Could you check a few things on this model? Use its own coordinates, in mm. Face numbers are marked on the shaded views. A direction names the side the tool comes from. Give positions to 0.01 mm unless a question says otherwise; leave off trailing zeros. Write each loop counter-clockwise with the first axis right and the second up, starting at its lowest first coordinate (ties: lowest second). Pieces come first, ordered by that corner, then holes. Notation, with made-up numbers: M -23.75,39.25 L 28.25,39.25 A9 ccw 28.25,47.25 Z; hole C 69.5,-6 d1. An arc over 180 degrees is marked long. Use one line per item in the form item = value.
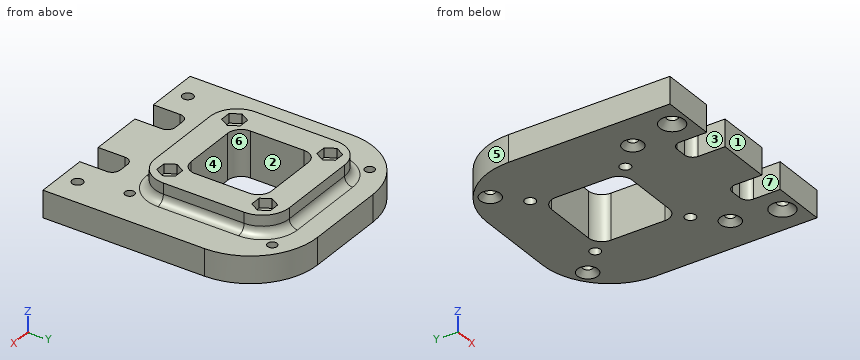
Autodesk Inventor part; units mm, degrees
ref_plane "YZ Plane" through (0, 0, 0) normal (1, 0, 0) x (0, 1, 0)
ref_plane "XZ Plane" through (0, 0, 0) normal (0, 1, 0) x (-1, 0, 0)
ref_plane "XY Plane" through (0, 0, 0) normal (0, 0, 1) x (1, 0, 0)
sketch "Sketch1" plane through (0, 0, 0) normal (0, 0, 1) x (1, 0, 0)
  line L0 (10.3456, 14.8047) -> (30.3456, 14.8047)
  line L1 (40.3456, 14.8047) -> (60.3456, 14.8047)
  line L2 (70.3456, 14.8047) -> (90.3456, 14.8047)
  circle A0 centre (20.3456, 20.8047) radius 2
  circle A1 centre (80.3456, 20.8047) radius 2
  circle A2 centre (23.8456, 90.8047) radius 1.75
  circle A3 centre (76.8456, 90.8047) radius 1.75
  circle A4 centre (76.8456, 37.8047) radius 1.75
  circle A5 centre (23.8456, 37.8047) radius 1.75
  arc A6 (75.3456, 79.3047) -> (65.3456, 89.3047) centre (65.3456, 79.3047) ccw
  arc A7 (35.3456, 89.3047) -> (25.3456, 79.3047) centre (35.3456, 79.3047) ccw
  arc A8 (65.3456, 39.3047) -> (75.3456, 49.3047) centre (65.3456, 49.3047) ccw
  arc A9 (25.3456, 49.3047) -> (35.3456, 39.3047) centre (35.3456, 49.3047) ccw
  arc A10 (40.3456, 79.3047) -> (35.3456, 74.3047) centre (40.3456, 74.3047) ccw
  arc A11 (65.3456, 74.3047) -> (60.3456, 79.3047) centre (60.3456, 74.3047) ccw
  arc A12 (35.3456, 54.3047) -> (40.3456, 49.3047) centre (40.3456, 54.3047) ccw
  arc A13 (60.3456, 49.3047) -> (65.3456, 54.3047) centre (60.3456, 54.3047) ccw
  arc A14 (33.3456, 27.8047) -> (30.3456, 24.8047) centre (33.3456, 24.8047) ccw
  arc A15 (40.3456, 24.8047) -> (37.3456, 27.8047) centre (37.3456, 24.8047) ccw
  arc A16 (63.3456, 27.8047) -> (60.3456, 24.8047) centre (63.3456, 24.8047) ccw
  arc A17 (70.3456, 24.8047) -> (67.3456, 27.8047) centre (67.3456, 24.8047) ccw
  line L3 (34.668, 78.5182) -> (36.668, 81.9823)
  line L4 (34.668, 85.4464) -> (30.668, 85.4464)
  line L5 (28.668, 81.9823) -> (30.668, 78.5182)
  line L6 (70.0233, 78.5182) -> (72.0233, 81.9823)
  line L7 (70.0233, 85.4464) -> (66.0233, 85.4464)
  line L8 (64.0233, 81.9823) -> (66.0233, 78.5182)
  line L9 (70.0233, 43.1629) -> (72.0233, 46.627)
  line L10 (70.0233, 50.0911) -> (66.0233, 50.0911)
  line L11 (64.0233, 46.627) -> (66.0233, 43.1629)
  line L12 (34.668, 43.1629) -> (36.668, 46.627)
  line L13 (34.668, 50.0911) -> (30.668, 50.0911)
  line L14 (28.668, 46.627) -> (30.668, 43.1629)
  arc A18 (35.3456, 99.8047) -> (10.3456, 74.8047) centre (35.3456, 74.8047) ccw
  arc A19 (90.3456, 74.8047) -> (65.3456, 99.8047) centre (65.3456, 74.8047) ccw
  line L15 (10.3456, 74.8047) -> (10.3456, 14.8047)
  line L16 (30.3456, 14.8047) -> (30.3456, 24.8047)
  line L17 (33.3456, 27.8047) -> (37.3456, 27.8047)
  line L18 (40.3456, 14.8047) -> (40.3456, 24.8047)
  line L19 (60.3456, 14.8047) -> (60.3456, 24.8047)
  line L20 (63.3456, 27.8047) -> (67.3456, 27.8047)
  line L21 (70.3456, 24.8047) -> (70.3456, 14.8047)
  line L22 (90.3456, 14.8047) -> (90.3456, 74.8047)
  line L23 (35.3456, 99.8047) -> (65.3456, 99.8047)
  line L24 (35.3456, 89.3047) -> (65.3456, 89.3047)
  line L25 (75.3456, 79.3047) -> (75.3456, 49.3047)
  line L26 (65.3456, 39.3047) -> (35.3456, 39.3047)
  line L27 (25.3456, 49.3047) -> (25.3456, 79.3047)
  line L28 (30.668, 85.4464) -> (28.668, 81.9823)
  line L29 (34.668, 85.4464) -> (36.668, 81.9823)
  line L30 (34.668, 78.5182) -> (30.668, 78.5182)
  line L31 (64.0233, 81.9823) -> (66.0233, 85.4464)
  line L32 (70.0233, 85.4464) -> (72.0233, 81.9823)
  line L33 (70.0233, 78.5182) -> (66.0233, 78.5182)
  line L34 (30.668, 50.0911) -> (28.668, 46.627)
  line L35 (30.668, 43.1629) -> (34.668, 43.1629)
  line L36 (36.668, 46.627) -> (34.668, 50.0911)
  line L37 (64.0233, 46.627) -> (66.0233, 50.0911)
  line L38 (70.0233, 50.0911) -> (72.0233, 46.627)
  line L39 (70.0233, 43.1629) -> (66.0233, 43.1629)
  circle A20 centre (32.668, 81.9823) radius 2
  circle A21 centre (68.0233, 81.9823) radius 2
  circle A22 centre (68.0233, 46.627) radius 2
  circle A23 centre (32.668, 46.627) radius 2
  line L40 (35.3456, 74.3047) -> (35.3456, 54.3047)
  line L41 (40.3456, 49.3047) -> (60.3456, 49.3047)
  line L42 (65.3456, 54.3047) -> (65.3456, 74.3047)
  line L43 (60.3456, 79.3047) -> (40.3456, 79.3047)
  point P0 (0, 0)
  dimension "d0" = 4
  dimension "d1" = 4
  dimension "d2" = 4
  dimension "d3" = 4
extrude "Extrusion1" add sketch "Sketch1" along normal blind 10 contours L15 A18 L23 A19 L22 L2 L21 A17 L20 A16 L19 L1 L18 A15 L17 A14 L16 L0
extrude "Extrusion3" add sketch "Sketch1" along normal blind 17 contours L25 A8 L26 A9 L27 A7 L24 A6
extrude "Extrusion4" add sketch "Sketch1" along normal blind 13.5 contours L30 L5 L28 L4 L29 L3 | L33 L8 L31 L7 L32 L6 | L39 L11 L37 L10 L38 L9 | L35 L14 L34 L13 L36 L12
fillet "Fillet1" radius 3 8 edges at (72.4167, 42.2336, 10) (50.3456, 39.3047, 10) (28.2746, 42.2336, 10) (25.3456, 64.3047, 10) (28.2746, 86.3757, 10) (50.3456, 89.3047, 10) (72.4167, 86.3757, 10) (75.3456, 64.3047, 10)
chamfer "Chamfer1" distance 2 angle 45 4 edges at (75.0956, 90.8047, 0) (22.0956, 90.8047, 0) (75.0956, 37.8047, 0) (22.0956, 37.8047, 0)
chamfer "Chamfer2" distance 2.5 angle 45 2 edges at (78.3456, 20.8047, 0) (18.3456, 20.8047, 0)
properties part number "mbot_rear_UTM-30LX_mount"
1) I want a section at B-B, the plane y = 58. Please give me the cut outline in (x, z).
Checked values:
outline = M 10.35,0 L 35.35,0 L 35.35,17 L 25.35,17 L 25.35,13 A3 cw 22.35,10 L 10.35,10 Z; M 65.35,0 L 90.35,0 L 90.35,10 L 78.35,10 A3 cw 75.35,13 L 75.35,17 L 65.35,17 Z
2) For the marked faces 1, 2 and 3, which set-ups out of +Z, -Z, +X, -X, +Y, -Y let a thin tool reach every point of the face, with its end or its side?
Checked values:
face_1 = +Z, -Z, +X, -X, -Y
face_2 = +Z, -Z
face_3 = +Z, -Z, -Y
3) Thinking about a two-plate mould opening in Y: for the marked faces 4, 5, 6 and 7, which applies, released by +Y, released by -Y, zero draft, split by the parting line, or undercut?
Checked values:
face_4 = undercut
face_5 = released by +Y
face_6 = undercut
face_7 = zero draft
4) For pin 1 Ø4.5 at (x, z) = (48, 15) entering from -Y; pin 2 Ø1 at (x, z) = (68, 14.5) entering from -Y; pin 3 Ø3 at (y, z) = (57, 14.5) entering from +X, each with a flat end and sliding along its axis, tell me the tip position at first contact or that it passes through.
Checked values:
pin_1 = 39.29
pin_2 = 39.54
pin_3 = 75.35
5) I want a section at C-C, the plane z = 15. Count the separate pieces of the cut face and the enclosed holes in it, plus the area to 3 significant figures.
Checked values:
separate_pieces = 1
enclosed_holes = 5
area = 1,370 mm2
6) If I drill on L1, parallel to X at y = 90.5, z = 4.25; L2, parallel to X at y = 20, z = 3; L3, parallel to X at y = 64.5, z = 3.25, over which ranges is the centre line in solid material (lowest first)?
Checked values:
L1 = 15.89 to 22.12, 25.57 to 75.12, 78.57 to 84.8
L2 = 10.35 to 18.51, 22.18 to 30.35, 40.35 to 60.35, 70.35 to 78.51, 82.18 to 90.35
L3 = 10.35 to 35.35, 65.35 to 90.35
7) I want a section at A-A, the plane x = 51. Please give me the cut outline in (y, z).
Checked values:
outline = M 14.8,0 L 49.3,0 L 49.3,17 L 39.3,17 L 39.3,13 A3 cw 36.3,10 L 14.8,10 Z; M 79.3,0 L 99.8,0 L 99.8,10 L 92.3,10 A3 cw 89.3,13 L 89.3,17 L 79.3,17 Z
